Source: CAD feature listing. Evaluate the final solid. Frame: model axes, mm. A direction names the side the tool comes from. Round coordinates to 2 decimals unless told otherwise and drop trailing zeros. Order: outer loops, then holes, each group sorted by start corner. A loop starts at its lowest first (then second) coordinate and runs counter-clockwise, first axis right, second up. Notation, with made-up numbers: M 7,-6.5 L 60,-6.5 A11 ccw 60,1.5 Z; hole C 36,-20 d6. An arc over 180 degrees is marked long. Answer in a Markdown table with one row per item. Add a question column.
```python
from build123d import *

# Parameters (mm, degrees)
F0_R     = 31
F0_R_2   = 28.75
F0_R_3   = 27.1
F0_R_4   = 25.6
F1_DEPTH = 3
F2_DEPTH = 10
F3_DEPTH = 3
F4_DEPTH = 25
F5_SIZE  = 0.5


with BuildPart() as f1:
    # F0 (on Top) → F1 (new body)
    with BuildSketch(Plane.XY):
        Circle(F0_R)
        Circle(F0_R_2, mode=Mode.SUBTRACT)
        Circle(F0_R_2)
        Circle(F0_R_3, mode=Mode.SUBTRACT)
        Circle(F0_R_3)
        Circle(F0_R_4, mode=Mode.SUBTRACT)
    extrude(amount=-F1_DEPTH)

    # F0 (on Top) → F2 (join)
    with BuildSketch(Plane.XY):
        Circle(F0_R_3)
        Circle(F0_R_4, mode=Mode.SUBTRACT)
    extrude(amount=F2_DEPTH)

    # F0 (on Top) → F3 (join)
    with BuildSketch(Plane.XY):
        Circle(F0_R)
        Circle(F0_R_2, mode=Mode.SUBTRACT)
    extrude(amount=F3_DEPTH)

    # F0 (on Top) → F4 (cut)
    with BuildSketch(Plane.XY):
        Circle(F0_R_4)
    extrude(amount=F4_DEPTH, mode=Mode.SUBTRACT)

    # F5
    f5_edges = [f1.edges().sort_by_distance(p)[0] for p in [
        (-25.6, 0, 10),
        (-27.1, 0, 10),
        (-28.75, 0, 3),
        (-25.6, 0, -3),
        (-31, 0, -3),
    ]]
    chamfer(f5_edges, length=F5_SIZE)


solid = f1.part
```
(1) Cut plane D-D (z = 5.25). Return loops of the section in (x, y).
(2) Pin query (flat end, axial travel): pin 1 (2 mm diameter, centred on x = -20, z = 6.5, fed in from -Y); pin 2 (1 mm diameter, centred on x = -20.5, z = 3, fed in from -Y); pin 3 (5 mm diameter, centred on x = -7, z = -1, fed in from -Y). Return the tip coordinate at first contact, or that it passes through.
(3) Cut plane C-C (z = -1.5). Return loops of the section in (x, y).
(4) Cut plane A-A (x = 0). Return loops of the section in (y, z), and give its area (4 significant figures).
(5) Line query: line 1 (Y direction, x = 0, z = 1); line 2 (Y direction, x = 21.5, z = 0.25); line 3 (Y direction, x = 0.5, z = 8.75). Output: solid intervals per line, ascending. Write a range as from..to.
(6) Draft query along X for faces 3 (the face through (23, 19, 3)), 4 (the face through (-6.232, -28.066, 1.232)), 5 (the face through (-4.036, 30.736, 0.288)). Return one class per face: +X half, -X half, draft (parallel to the pull), parting line (faces both ways), or undercut.
(7) Access query for faces 1 (the face through (-9, 26, 0)), 2 (the face through (19.6, -17.6, 10)). Directions: +Z, -Z, +X, -X, +Y, -Y. A direction counts if a zero-diameter tool reaches every point of the face in a straight line with its end or side. Return the directions, or none.
Answer list:
| question | item | result |
|---|---|---|
| 1 | outline | C 0,0 d54.2; hole C 0,0 d51.2 |
| 2 | pin 1 | y = -19.32 |
| 2 | pin 2 | y = -23.69 |
| 2 | pin 3 | y = -30.67 |
| 3 | outline | C 0,0 d62; hole C 0,0 d51.2 |
| 4 | outline | M -31,-2.5 L -30.5,-3 L -26.1,-3 L -25.6,-2.5 L -25.6,9.5 L -26.1,10 L -26.6,10 L -27.1,9.5 L -27.1,0 L -28.75,0 L -28.75,2.5 L -29.25,3 L -31,3 Z; M 25.6,-2.5 L 26.1,-3 L 30.5,-3 L 31,-2.5 L 31,3 L 29.25,3 L 28.75,2.5 L 28.75,0 L 27.1,0 L 27.1,9.5 L 26.6,10 L 26.1,10 L 25.6,9.5 Z |
| 4 | area | 74.65 mm² |
| 5 | line 1 | -31..-28.75, -27.1..-25.6, 25.6..27.1, 28.75..31 |
| 5 | line 2 | -22.33..-19.09, -16.5..-13.9, 13.9..16.5, 19.09..22.33 |
| 5 | line 3 | -27.1..-25.6, 25.6..27.1 |
| 6 | face 3 | draft |
| 6 | face 4 | undercut |
| 6 | face 5 | parting line |
| 7 | face 1 | +Z |
| 7 | face 2 | +Z, +X, -X, +Y, -Y |
